from build123d import *

# Parameters (mm, degrees)
SKETCH1_W           = 46
SKETCH1_H           = 46
SKETCH1_R           = 2
BOSS_EXTRUDE1_DEPTH = 1.5
BOSS_EXTRUDE2_DEPTH = 12
FILLET1_R           = 1
SKETCH4_R           = 1.5
BOSS_EXTRUDE3_DEPTH = 4.52
FILLET2_R           = 10


with BuildPart() as part:
    # Sketch1 → Boss-Extrude1 (new body)
    with BuildSketch(Plane.XY):
        Rectangle(SKETCH1_W, SKETCH1_H)
        with Locations((0, 7)):
            Circle(SKETCH1_R, mode=Mode.SUBTRACT)
    extrude(amount=BOSS_EXTRUDE1_DEPTH)

    # Sketch3 → Boss-Extrude2 (add)
    with BuildSketch(Plane(origin=(0, 0, 0), x_dir=(-1, 0, 0), z_dir=(0, 0, -1))):
        with BuildLine():
            Line((16.045296796, -5.501477845), (13.954703204, -5.501477845))
            ThreePointArc((13.954703204, -5.501477845), (11.306350983, -9.857303254), (7.352141129, -13.074632722))
            ThreePointArc((7.352141129, -13.074632722), (0, -15), (-7.352141129, -13.074632722))
            ThreePointArc((-7.352141129, -13.074632722), (-9.857303254, 11.306350983), (13.954703204, 5.501477845))
            Line((13.954703204, 5.501477845), (16.045296796, 5.501477845))
            Line((16.045296796, 5.501477845), (16.045296796, -5.501477845))
        make_face()
    extrude(amount=BOSS_EXTRUDE2_DEPTH)

    # Fillet1
    fillet1_edges = [part.edges().sort_by_distance(p)[0] for p in [
        (15, 0, -12),
    ]]
    fillet(fillet1_edges, radius=FILLET1_R)

    # Sketch4 → Boss-Extrude3 (add)
    with BuildSketch(Plane.XY):
        with Locations((0, 7)):
            Circle(SKETCH4_R)
    extrude(amount=BOSS_EXTRUDE3_DEPTH)

    # Fillet2
    fillet2_edges = [part.edges().sort_by_distance(p)[0] for p in [
        (23, -23, 0.75),
        (-23, -23, 0.75),
        (-23, 23, 0.75),
        (23, 23, 0.75),
    ]]
    fillet(fillet2_edges, radius=FILLET2_R)


solid = part.part
Could you check a few things on this model? Use its own coordinates, in mm. A direction names the side the tool comes from. Give positions to 0.01 mm unless a question says otherwise; leave off trailing zeros. Order: outer loops, then holes, each group sorted by start corner. A loop starts at its lowest first (then second) coordinate and runs counter-clockwise, first axis right, second up.
1. For pin 1 (2.5 mm diameter, centred on x = -15, z = -8.5, fed in from +Y); pin 2 (1.5 mm diameter, centred on x = -8.5, z = -5, fed in from -Y); pin 3 (1 mm diameter, centred on y = 9, z = -2, fed in from +X), each with a flat end and sliding along its axis, tell me the tip position at first contact or that it passes through.
Answers below:
pin 1: stops at y = 5.99
pin 2: stops at y = -12.84
pin 3: stops at x = 12.36
2. Suppose I cut it at B-B (z = 3.75). Write out the boundary of the cut face in (x, y), plus the area to 3 significant figures.
Answers below:
outline: circle Ø3 at (0, 7)
area: 7.07 mm2
3. Suppose I cut it at A-A (z = -9). Write out the boundary of the cut face in (x, y), plus the area to 3 significant figures.
Answers below:
outline: (-16.05, -5.5) - (-13.95, -5.5) arc R15 ccw (long way) to (-13.95, 5.5) - (-16.05, 5.5) - close
area: 722 mm2
4. I need wall thicknesses on L1, parallel to Y at x = 0, z = 0.4; L2, parallel to Z at x = 18.5, y = 17; L3, parallel to Z at x = 4, y = 8.5. Which ranges of each line are inside material? Lowest first, please.
Answers below:
L1: y = -23 to 5, 5.5 to 8.5, 9 to 23
L2: z = 0 to 1.5
L3: z = -12 to 1.5
5. Thinking about a two-plate mould opening in Y: for faces 1 (the cylindrical face through (-0.325, 5.536, 2.228)), 2 (the flat face through (0, 0, 1.5)), 3 (the flat face through (-15, -5.501, -6)), which applies, +Y half, -Y half, draft (parallel to the pull), parting line (faces both ways), or undercut?
Answers below:
face 1: undercut
face 2: draft
face 3: -Y half
6. Which directions (+Z, -Z, +X, -X, +Y, -Y) give clear straight access to the entire face, cutting with the end or side of a thin tool? Please do faces 4 (the flat face through (-15, 5.501, -6)), 5 (the flat face through (-16.045, 0, -6)), 6 (the cylindrical face through (-20.15, 19.99, 0.76)), 7 (the flat face through (15, -5, 0)), 8 (the cylindrical face through (0, 9, 1)).
Answers below:
face 4: -Z, -X, +Y
face 5: -Z, -X, +Y, -Y
face 6: +Z, -Z, -X, +Y
face 7: -Z
face 8: +Z
